The listing builds one solid part. Answer for the finished solid, in the listing's coordinates (mm). A direction names the side the tool comes from. Round coordinates to 2 decimals unless told otherwise and drop trailing zeros. Write each loop counter-clockwise with the first axis right and the second up, starting at its lowest first coordinate (ties: lowest second). Pieces come first, ordered by that corner, then holes. Notation, with made-up numbers: M 36.5,20 L 65.5,20 A20 cw 65.5,53 Z; hole C -20,75.5 d7. An arc over 180 degrees is marked long. One line per item, written item: value. Start each with the question number.
(1) For a pull along X with two mould halves and no side action, classify faces 1 (the flat face through (38, 73, 0)), 2 (the flat face through (0, 37, 2)), 3 (the cylindrical face through (5.2, 4.05, 2.46)) as released by +X, released by -X, zero draft, split by the parting line, or undercut.
(2) Section A-A (x = 66) is taken. Determine the outline of the cut face in (y, z), plus the area to 3 significant figures.
(3) Section D-D (y = 4) is taken. Determine the outline of the cut face in (x, z).
(4) For faces 4 (the flat face through (8, 33, 2)), 5 (the flat face through (80, 70, 2)), 6 (the cylindrical face through (64.89, 3.54, 2.46)), determine the directions among +Z, -Z, +X, -X, +Y, -Y from which every point of the face is accessible in a straight line to the end or side of a thin tool.
(5) Section C-C (y = 60) is taken. Determine the outline of the cut face in (x, z).
(6) Section B-B (z = 1.9) is taken. Determine the outline of the cut face in (x, y), plus the area to 3 significant figures.
(7) Consider probe 1 along X at (y, z) = (4, 1.6); probe 2 along X at (y, z) = (52, 3.75); probe 3 along Y at (x, z) = (66, 3.2). Determine where each line is inside the solid, lowest interval first.
```python
from build123d import *

# Parameters (mm, degrees)
ESQUISSE1_R          = 1
BOSS_EXTRU_1_DEPTH   = 5
D_GAGEMENT_M21_D     = 2.4
D_GAGEMENT_M21_DEPTH = 5
D_GAGEMENT_M21_TIP   = 0.721032743
CONG_1_START         = -1
CONG_1_DEPTH         = 7
CONG_1_2_DEPTH       = 5


with BuildPart() as part:
    # Esquisse1 → Boss.-Extru.1 (new body)
    with BuildSketch(Plane.XY):
        Polygon((0, 0), (0, 80), (90, 80), (90, 70), (70, 70), (70, 0), (62, 0), (62, 70), (8, 70), (8, 0), align=None)
        with Locations((4, 4)):
            Circle(ESQUISSE1_R, mode=Mode.SUBTRACT)
        with Locations((66, 4)):
            Circle(ESQUISSE1_R, mode=Mode.SUBTRACT)
    extrude(amount=BOSS_EXTRU_1_DEPTH)

    # Dégagement M21
    with Locations(Plane.XY.offset(5)):
        with Locations((4, 4), (66, 4)):
            Hole(D_GAGEMENT_M21_D / 2, depth=D_GAGEMENT_M21_DEPTH)
            with Locations((0, 0, -(D_GAGEMENT_M21_DEPTH + D_GAGEMENT_M21_TIP / 2))):  # 118° drill point
                Cone(0, D_GAGEMENT_M21_D / 2, D_GAGEMENT_M21_TIP, mode=Mode.SUBTRACT)

    # Congé1: read off the stored shape, not the designer's step
    # Congé1 outline → Congé1 (cut)
    with BuildSketch(Plane.XY.offset(CONG_1_START)):
        with BuildLine():
            Line((0, 80), (0, 75))
            ThreePointArc((0, 75), (1.464466094, 78.535533906), (5, 80))
            Line((5, 80), (0, 80))
        make_face()
        with BuildLine():
            Line((90, 70), (90, 75))
            ThreePointArc((90, 75), (88.535533906, 71.464466094), (85, 70))
            Line((85, 70), (90, 70))
        make_face()
        with BuildLine():
            Line((90, 80), (85, 80))
            ThreePointArc((85, 80), (88.535533906, 78.535533906), (90, 75))
            Line((90, 75), (90, 80))
        make_face()
    extrude(amount=CONG_1_DEPTH, mode=Mode.SUBTRACT)

    # Cong_1 2 outline → Cong_1 2 (add)
    with BuildSketch(Plane.XY):
        with BuildLine():
            ThreePointArc((70, 65), (71.464466094, 68.535533906), (75, 70))
            Line((75, 70), (70, 70))
            Line((70, 70), (70, 65))
        make_face()
        with BuildLine():
            ThreePointArc((8, 65), (9.464466094, 68.535533906), (13, 70))
            Line((13, 70), (8, 70))
            Line((8, 70), (8, 65))
        make_face()
        with BuildLine():
            ThreePointArc((57, 70), (60.535533906, 68.535533906), (62, 65))
            Line((62, 65), (62, 70))
            Line((62, 70), (57, 70))
        make_face()
    extrude(amount=CONG_1_2_DEPTH)


solid = part.part
```
Recorded:
1. face 1: zero draft
1. face 2: released by -X
1. face 3: undercut
2. outline: M 0,0 L 2.8,0 L 2.8,5 L 0,5 Z; M 5.2,0 L 80,0 L 80,5 L 5.2,5 Z
2. area: 388 mm2
3. outline: M 0,0 L 2.8,0 L 2.8,5 L 0,5 Z; M 5.2,0 L 8,0 L 8,5 L 5.2,5 Z; M 62,0 L 64.8,0 L 64.8,5 L 62,5 Z; M 67.2,0 L 70,0 L 70,5 L 67.2,5 Z
4. face 4: +Z, -Z, -Y
4. face 5: +Z, -Z, +X, -Y
4. face 6: +Z, -Z
5. outline: M 0,0 L 8,0 L 8,5 L 0,5 Z; M 62,0 L 70,0 L 70,5 L 62,5 Z
6. outline: M 0,0 L 8,0 L 8,65 A5 cw 13,70 L 57,70 A5 cw 62,65 L 62,0 L 70,0 L 70,65 A5 cw 75,70 L 85,70 A5 ccw 85,80 L 5,80 A5 ccw 0,75 Z; hole C 4,4 d2.4; hole C 66,4 d2.4
6. area: 2,010 mm2
7. probe 1: x = 0 to 2.8, 5.2 to 8, 62 to 64.8, 67.2 to 70
7. probe 2: x = 0 to 8, 62 to 70
7. probe 3: y = 0 to 2.8, 5.2 to 80
